Geometry check sheet. Reference: the model listing, model coordinates, mm. Give positions to 0.01 mm unless a question says otherwise; leave off trailing zeros. Order: outer loops, then holes, each group sorted by start corner. A loop starts at its lowest first (then second) coordinate and runs counter-clockwise, first axis right, second up. Notation, with made-up numbers: M 78.5,52 L 85.5,52 A15 ccw 85.5,79 Z; hole C 50,-19.5 d8. An arc over 180 degrees is marked long. Put each result on its own line as item: value. Start each with the question number.
Q1. Material ranges on L1, parallel to Z at x = 0.5, y = -4.5; L2, parallel to X at y = 4.5, z = 0.65; L3, parallel to Y at x = -0.5, z = 0.4, recorded low to high.
Q2. Section check A-A on x = 0. Record the cut outline in (y, z), then the cut area to 3 significant figures.
Q3. Go/stop test with flat-tipped pins: pin 1 (4 mm diameter, centred on x = -10.5, y = 1, fed in from +Z); pin 2 (5 mm diameter, centred on x = -6.5, y = 2.5, fed in from -Z); pin 3 (0.6 mm diameter, centred on x = -0.5, z = 1, fed in from -Y). Record where each tip stops, or that it passes through.
Q4. Section check D-D on y = 7.5. Record the cut outline in (x, z).
Q5. Section check B-B on y = 0. Record the cut outline in (x, z), then the cut area to 3 significant figures.
Q6. Section check C-C on z = 0.7. Record the cut outline in (x, y), then the cut area to 3 significant figures.
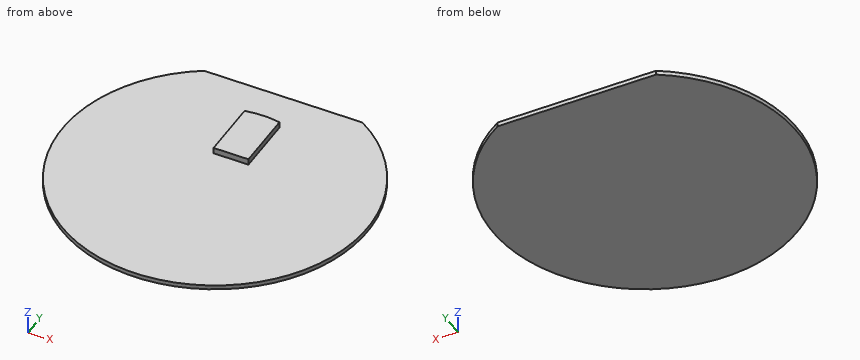
Autodesk Fusion 360 part; units mm, degrees
sketch "Szkic1" plane through (0, 0, 0) normal (0, 0, 1) x (1, 0, 0)
  circle A0 centre (0, 0) radius 10.5
  line L0 (0, 10.5) -> (0, 3.5) construction
  line L1 (0, 3.5) -> (2, 3.5)
  line L2 (2, 3.5) -> (2, 11)
  line L3 (2, 11) -> (-2, 11)
  line L4 (-2, 11) -> (-2, 3.5)
  line L5 (-2, 3.5) -> (0, 3.5)
  circle A1 centre (0, 0) radius 17.5
  line L6 (9.089, 14.9546) -> (-9.089, 14.9546)
  dimension "d1" = 21
  dimension "d2" = 7
  dimension "d3" = 2
  dimension "d4" = 3.5
  dimension "d5" = 2
  dimension "d6" = 3.5
  dimension "d7" = 0.5
  dimension "d10" = 35
  dimension "d15" = 18.1779
extrude "Wyciągnięcie proste1" add sketch "Szkic1" along normal blind 1 contours A0 L1 L2 L4 L5 picked at (-1.3333, 5.7693)
extrude "Wyciągnięcie proste2" add sketch "Szkic1" along normal blind 0.5 contours A0 L1 L2 L4 L5 | A0 L2 L3 L4 | A1 L6 picked at (1.5608, -1.0505) picked at (0.6667, 13.6364)
extrude "Wyciągnięcie proste3" add 1 faces at (-0.2234, 5.8262, 1) along direction (0, 0, 1) blind 0.2
Results found:
1. L1: z = 0 to 0.5
1. L2: x = -2 to 2
1. L3: y = -17.49 to 14.95
2. outline: M -17.5,0 L 14.95,0 L 14.95,0.5 L 10.5,0.5 L 10.5,1.2 L 3.5,1.2 L 3.5,0.5 L -17.5,0.5 Z
2. area: 21.1 mm^2
3. pin 1: stops at z = 0.5
3. pin 2: stops at z = 0
3. pin 3: stops at y = 3.5
4. outline: M -15.81,0 L 15.81,0 L 15.81,0.5 L 2,0.5 L 2,1.2 L -2,1.2 L -2,0.5 L -15.81,0.5 Z
5. outline: M -17.5,0 L 17.5,0 L 17.5,0.5 L -17.5,0.5 Z
5. area: 17.5 mm^2
6. outline: M -2,3.5 L 2,3.5 L 2,10.31 A10.5 ccw -2,10.31 Z
6. area: 27.7 mm^2
